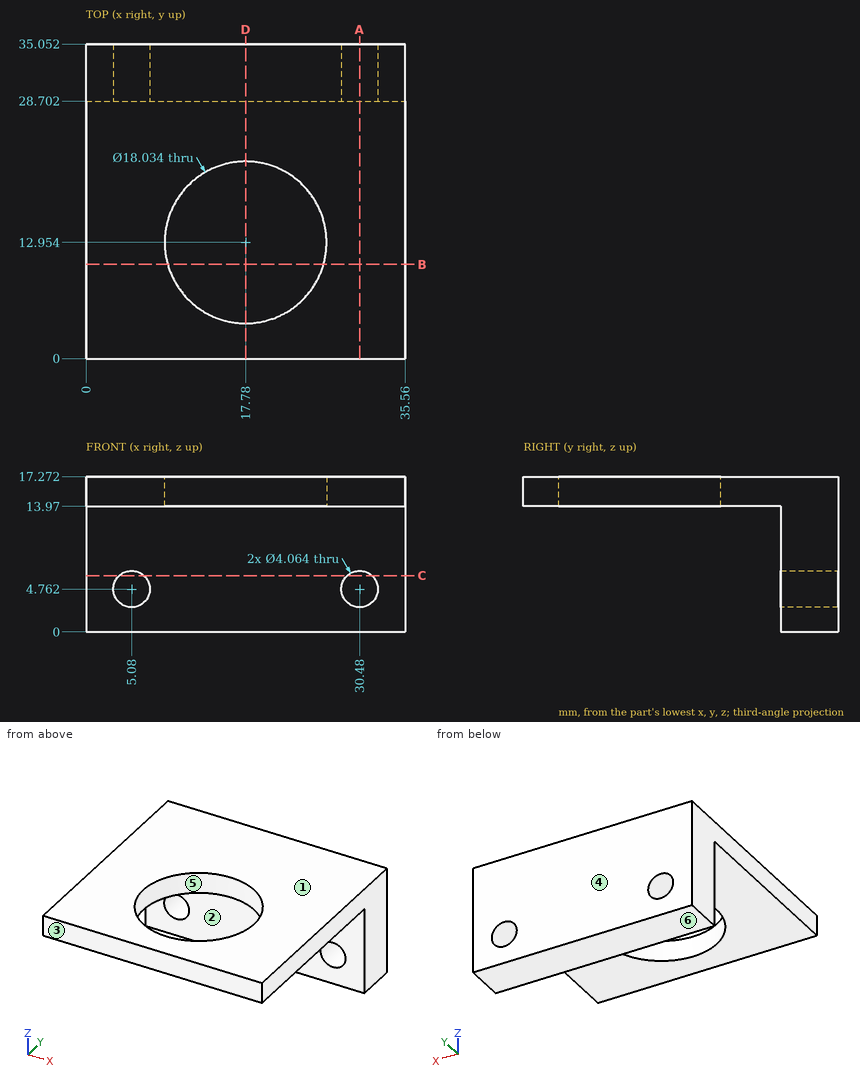
Check sheet for the drawn part. Datum: minimum x, y, z corner. Units: mm. A direction names the side the tool comes from. Coordinates: 2 decimals unless noted, no trailing zeros. Order: outer loops, then holes, each group sorted by start corner. A loop starts at its lowest first (then second) coordinate and runs counter-clockwise, first axis right, second up. Notation, with made-up numbers: (-14, 81) -> (22, 81) arc R24 ccw to (22, 114) -> close; hole circle Ø11 at (6.25, -3). An arc over 180 degrees is marked (long way). Use a Markdown table: item, result. Add a question column.
1. Cross-section at D-D (x = 17.78). Enter the section's corners in (y, z).
2. Set-up check for the marked faces 1 and 2: record each of +Z, -Z, +X, -X, +Y, -Y from which the full face is reachable in a straight line by a thin tool's end or side.
3. Mould release check, pull along Y, two halves, no side actions. Record for the marked faces 3, 4, 5 and 6: pulls with the +Y half, pulls with the -Y half, needs draft (parallel to the pull), parting line crosses it, or undercut.
4. Cross-section at C-C (z = 6.25). Enter the section's corners in (x, y) (1 decimal).
5. Material ranges on L1, parallel to Y at x = 17.78, z = 15.9; L2, parallel to Y at x = 14.5, z = 11.5; L3, parallel to Z at x = 12.5, y = 20.5, recorded low to high.
6. Cross-section at B-B (y = 10.5). Enter the section's corners in (x, z).
7. Cross-section at A-A (x = 30.48). Enter the section's corners in (y, z) (1 decimal).
8. Go/stop test with a flat-tipped pin: pin 1 Ø1 at (x, y) = (27.5, 26.5) entering from -Z. Record where the tip stops, or that it passes through.
Filled sheet:
| question | item | result |
|---|---|---|
| 1 | outline | (0, 13.97) -> (3.94, 13.97) -> (3.94, 17.27) -> (0, 17.27) -> close; (21.97, 13.97) -> (28.7, 13.97) -> (28.7, 0) -> (35.05, 0) -> (35.05, 17.27) -> (21.97, 17.27) -> close |
| 2 | face 1 | +Z, +X, -X, +Y, -Y |
| 2 | face 2 | -Z, +X, -X, -Y |
| 3 | face 3 | pulls with the -Y half |
| 3 | face 4 | pulls with the +Y half |
| 3 | face 5 | undercut |
| 3 | face 6 | needs draft |
| 4 | outline | (0, 28.7) -> (3.7, 28.7) -> (3.7, 35.1) -> (0, 35.1) -> close; (6.5, 28.7) -> (29.1, 28.7) -> (29.1, 35.1) -> (6.5, 35.1) -> close; (31.9, 28.7) -> (35.6, 28.7) -> (35.6, 35.1) -> (31.9, 35.1) -> close |
| 5 | L1 | 0 to 3.94, 21.97 to 35.05 |
| 5 | L2 | 28.7 to 35.05 |
| 5 | L3 | 13.97 to 17.27 |
| 6 | outline | (0, 13.97) -> (9.1, 13.97) -> (9.1, 17.27) -> (0, 17.27) -> close; (26.46, 13.97) -> (35.56, 13.97) -> (35.56, 17.27) -> (26.46, 17.27) -> close |
| 7 | outline | (0, 14) -> (28.7, 14) -> (28.7, 6.8) -> (35.1, 6.8) -> (35.1, 17.3) -> (0, 17.3) -> close; (28.7, 0) -> (35.1, 0) -> (35.1, 2.7) -> (28.7, 2.7) -> close |
| 8 | pin 1 | z = 13.97 |
